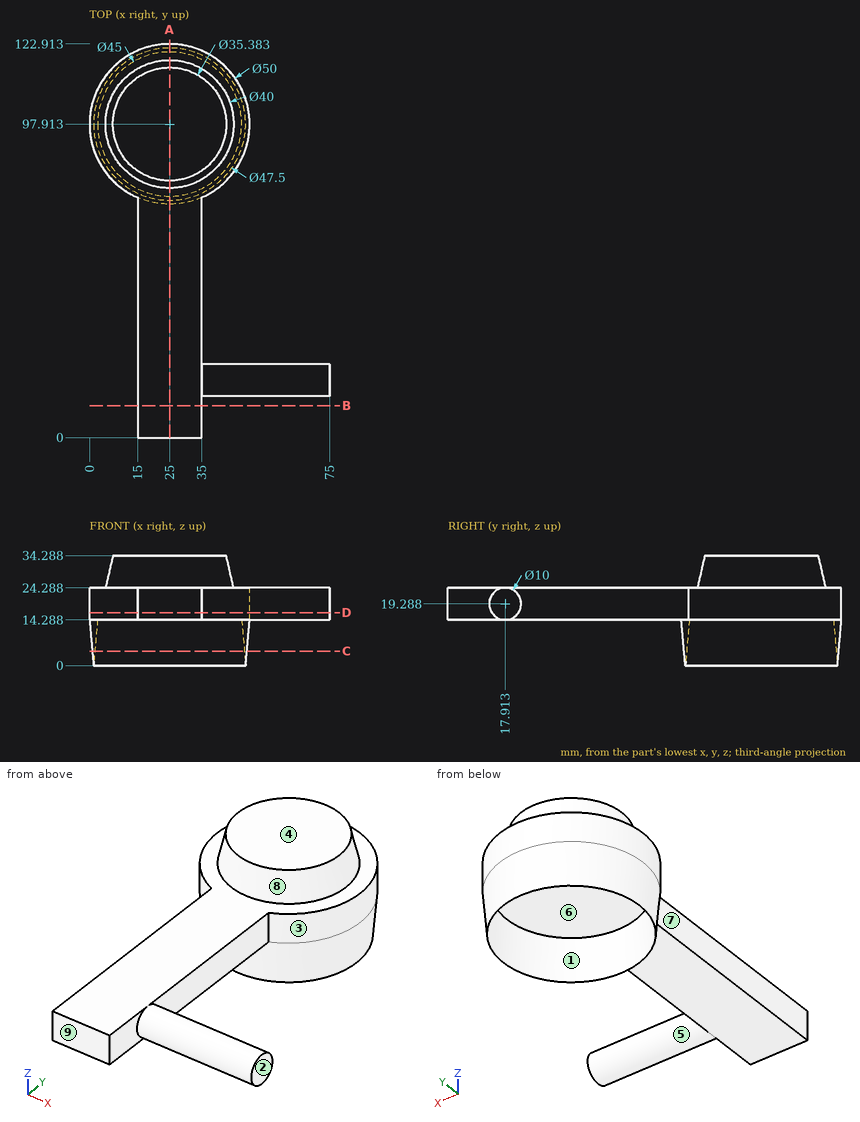
Geometry: see drawing. Coordinates: mm, zero at the bounding-box minimum. A direction names the side the tool comes from. Coordinates: 2 decimals unless noted, no trailing zeros. Write each loop counter-clockwise with the first axis right and the second up, starting at its lowest first coordinate (ties: lowest second). Pieces come first, ordered by that corner, then holes. Notation, with made-up numbers: M 40.25,67.25 L 68.25,67.25 A18 ccw 68.25,73.25 Z; hole C 1,-26 d5. An arc over 180 degrees is marked long. Answer as a JSON object with one key per item and string values.
1. Cut plane D-D on z = 16.5. Output: boundary loops of the cut face in (x, y).
Evaluation:
{"outline": "M 15,0 L 35,0 L 35,13.76 L 75,13.76 L 75,22.06 L 35,22.06 L 35,75 A25 ccw long 15,75 Z"}
2. Draft query along X for the marked faces 1, 2, 3 and 4. Return one class per face: released by +X, released by -X, zero draft, split by the parting line, or undercut.
Evaluation:
{"face 1": "undercut", "face 2": "released by +X", "face 3": "split by the parting line", "face 4": "zero draft"}
3. Cut plane B-B on y = 10. Output: boundary loops of the cut face in (x, z).
Evaluation:
{"outline": "M 15,14.29 L 35,14.29 L 35,24.29 L 15,24.29 Z"}
4. Ray query, L1, parallel to Z at x = 15.5, y = 116; L2, parallel to X at y = 96, z = 9; L3, parallel to X at y = 86, z = 4.5. Return the intervals inside material, ascending.
Evaluation:
{"L1": "14.29 to 24.29", "L2": "0.54 to 2.12, 47.88 to 49.46", "L3": "4 to 4.91, 45.09 to 46"}
5. Access query for the marked faces 5, 6, 7, 8 and 9. Directions: +Z, -Z, +X, -X, +Y, -Y. A direction counts if a zero-diameter tool reaches every point of the face in a straight line with its end or side. Return the directions, or none.
Evaluation:
{"face 5": "+X", "face 6": "-Z", "face 7": "+Z, -Z, -X, -Y", "face 8": "+Z", "face 9": "+Z, -Z, +X, -X, -Y"}
6. Cut plane A-A on x = 25. Output: boundary loops of the cut face in (y, z) (1 decimal), plus the area to 3 significant figures.
Evaluation:
{"outline": "M 0,14.3 L 72.9,14.3 L 74.2,0 L 75.4,14.3 L 120.4,14.3 L 121.7,0 L 122.9,14.3 L 122.9,24.3 L 117.9,24.3 L 115.6,34.3 L 80.2,34.3 L 77.9,24.3 L 0,24.3 Z", "area": "1,640 mm^2"}
7. Cut plane C-C on z = 4.5. Output: boundary loops of the cut face in (x, y).
Evaluation:
{"outline": "C 25,97.91 d48.29; hole C 25,97.91 d46.71"}
8. Contact query for flat-ended pins moving along their axis: P1, Ø8, axis at y = 37.5, z = 17, coming from the +X side; P2, Ø11, axis at y = 52.5, z = 18.5, coming from the -X side; P3, Ø2, axis at y = 110.5, z = 25, coming from the -X side (1 decimal). Output: stop coordinate, or through.
Evaluation:
{"P1": "x = 35", "P2": "x = 15", "P3": "x = 3"}
